Input: part model. Units: mm. Frame: model coordinates. A direction names the side the tool comes from. Give positions to 0.01 mm unless a question says otherwise; leave off trailing zeros. Loops run counter-clockwise (first coordinate to the right, second up) from the corner with the lowest first, then second, coordinate; pieces in that order, holes last. Notation, with made-up numbers: (-18.75, 45) -> (19.25, 45) arc R26 cw to (19.25, 72) -> close; hole circle Ø5 at (39, 75.25). An arc over 180 degrees is marked (long way). Answer as a JSON object with one key per item and string values.
```python
from build123d import *

# Parameters (mm, degrees)
SKETCH1_R           = 1.5
BOSS_EXTRUDE1_DEPTH = 1.6
SKETCH2_W           = 9.48
SKETCH2_H           = 4.83
BOSS_EXTRUDE2_DEPTH = 10
SKETCH3_R           = 2.65
SKETCH3_R_2         = 3.25
BOSS_EXTRUDE3_DEPTH = 12


with BuildPart() as part:
    # Sketch1 → Boss-Extrude1 (new body)
    with BuildSketch(Plane(origin=(0, 0, 0), x_dir=(1, 0, 0), z_dir=(0, 1, 0))):
        with BuildLine():
            Line((3.61, 0), (48.39, 0))
            ThreePointArc((48.39, 0), (50.94265548, 1.05734452), (52, 3.61))
            Line((52, 3.61), (52, 17.99))
            ThreePointArc((52, 17.99), (50.94265548, 20.54265548), (48.39, 21.6))
            Line((48.39, 21.6), (3.61, 21.6))
            ThreePointArc((3.61, 21.6), (1.05734452, 20.54265548), (0, 17.99))
            Line((0, 17.99), (0, 3.61))
            ThreePointArc((0, 3.61), (1.05734452, 1.05734452), (3.61, 0))
        make_face()
        with Locations(Location((3.61, 17.99, 0), (0, 0, 270))):
            Circle(SKETCH1_R, mode=Mode.SUBTRACT)
        with Locations(Location((48.39, 17.99, 0), (0, 0, 270))):
            Circle(SKETCH1_R, mode=Mode.SUBTRACT)
        with Locations(Location((48.39, 3.61, 0), (0, 0, 270))):
            Circle(SKETCH1_R, mode=Mode.SUBTRACT)
        with Locations(Location((3.61, 3.61, 0), (0, 0, 270))):
            Circle(SKETCH1_R, mode=Mode.SUBTRACT)
    extrude(amount=BOSS_EXTRUDE1_DEPTH)

    # Sketch2 → Boss-Extrude2 (add)
    with BuildSketch(Plane(origin=(0, 1.6, 0), x_dir=(1, 0, 0), z_dir=(0, 1, 0))):
        with Locations((19.47, 3.975)):
            Rectangle(SKETCH2_W, SKETCH2_H)
        with Locations((19.47, 18.795)):
            Rectangle(SKETCH2_W, SKETCH2_H)
    extrude(amount=BOSS_EXTRUDE2_DEPTH)

    # Sketch3 → Boss-Extrude3 (add)
    with BuildSketch(Plane(origin=(0, 1.6, 0), x_dir=(1, 0, 0), z_dir=(0, 1, 0))):
        with Locations(Location((35.19, 11, 0), (0, 0, 270))):
            Circle(SKETCH3_R)
        with Locations(Location((28.13, 13.6, 0), (0, 0, 270))):
            Circle(SKETCH3_R_2)
    extrude(amount=BOSS_EXTRUDE3_DEPTH)


solid = part.part
```
Q1. Pin query (flat end, axial travel): pin 1 (6 mm diameter, centred on y = 10.5, z = -17.5, fed in from -X); pin 2 (2.5 mm diameter, centred on x = 18.5, z = -3, fed in from +Y); pin 3 (1.5 mm diameter, centred on x = 21, y = 10, fed in from +Z); pin 4 (1.8 mm diameter, centred on x = 3.61, z = -17.99, fed in from +Y). Return the tip coordinate at first contact, or that it passes through.
Evaluation:
{"pin 1": "stops at x = 14.73", "pin 2": "stops at y = 11.6", "pin 3": "stops at z = -1.56", "pin 4": "passes through"}
Q2. Ray query, line 1 along X through (y, z) = (0.65, -17.99); line 2 along Z through (x, y) = (21, 4); line 3 along Y through (x, z) = (20, -1). Return the intervals inside material, ascending.
Evaluation:
{"line 1": "x = 0 to 2.11, 5.11 to 46.89, 49.89 to 52", "line 2": "z = -21.21 to -16.38, -6.39 to -1.56", "line 3": "y = 0 to 1.6"}
Q3. Draft query along Z for faces 1 (the flat face through (26, 1, -21.6)), 2 (the cylindrical face through (49.4, 0.8, -19.1)), 3 (the flat face through (24.21, 7, -4)). Return one class per face: +Z half, -Z half, draft (parallel to the pull), parting line (faces both ways), or undercut.
Evaluation:
{"face 1": "-Z half", "face 2": "undercut", "face 3": "draft"}
Q4. Section D-D, the plane z = -2.75. Return the cut outline in (x, y), then the cut area to 3 significant figures.
Evaluation:
{"outline": "(0.1, 0) -> (2.38, 0) -> (2.38, 1.6) -> (0.1, 1.6) -> close; (4.84, 0) -> (47.16, 0) -> (47.16, 1.6) -> (24.21, 1.6) -> (24.21, 11.6) -> (14.73, 11.6) -> (14.73, 1.6) -> (4.84, 1.6) -> close; (49.62, 0) -> (51.9, 0) -> (51.9, 1.6) -> (49.62, 1.6) -> close", "area": "170 mm2"}
Q5. Section C-C, the plane x = 35.19. Return the cut outline in (y, z).
Evaluation:
{"outline": "(0, -21.6) -> (1.6, -21.6) -> (1.6, -13.65) -> (13.6, -13.65) -> (13.6, -8.35) -> (1.6, -8.35) -> (1.6, 0) -> (0, 0) -> close"}
Q6. Access query for faces 4 (the flat face through (14.73, 7, -19)), 5 (the cylindrical face through (32.839, 7.516, -9.777)), 6 (the flat face through (19, 7, -21.21)), 7 (the flat face through (19, 7, -6.39)), 8 (the flat face through (19, 7, -16.38)). Directions: +Z, -Z, +X, -X, +Y, -Y. A direction counts if a zero-diameter tool reaches every point of the face in a straight line with its end or side. Return the directions, or none.
Evaluation:
{"face 4": "+Z, -Z, -X, +Y", "face 5": "+Y", "face 6": "-Z, +X, -X, +Y", "face 7": "+X, -X, +Y", "face 8": "-X, +Y"}
Q7. Section B-B, the plane y = 1. Return the cut outline in (x, z), then the cut area to 3 significant figures.
Evaluation:
{"outline": "(0, -17.99) arc R3.61 ccw to (3.61, -21.6) -> (48.39, -21.6) arc R3.61 ccw to (52, -17.99) -> (52, -3.61) arc R3.61 ccw to (48.39, 0) -> (3.61, 0) arc R3.61 ccw to (0, -3.61) -> close; hole circle Ø3 at (3.61, -17.99); hole circle Ø3 at (3.61, -3.61); hole circle Ø3 at (48.39, -17.99); hole circle Ø3 at (48.39, -3.61)", "area": "1,080 mm2"}
Q8. Section A-A, the plane y = 9. Return the cut outline in (x, z), then the cut area to 3 significant figures.
Evaluation:
{"outline": "(14.73, -21.21) -> (24.21, -21.21) -> (24.21, -16.38) -> (14.73, -16.38) -> close; (14.73, -6.39) -> (24.21, -6.39) -> (24.21, -1.56) -> (14.73, -1.56) -> close; circle Ø6.5 at (28.13, -13.6); circle Ø5.3 at (35.19, -11)", "area": "147 mm2"}
